CAD build for the part. Positions are in the model's coordinates, mm. A direction names the side the tool comes from. Give positions to 0.01 mm unless a question says otherwise; leave off trailing zeros. Loops run counter-clockwise (first coordinate to the right, second up) from the corner with the lowest first, then second, coordinate; pieces in that order, holes last.
Item 1: Which spindle directions (+Z, -Z, +X, -X, +Y, -Y) get a long thin tool onto all of the face, cutting with end or side? Do faces 4 (the flat face through (-24, 10.22, 1)), 5 (the flat face through (20, -9.12, 1)), 6 (the flat face through (0, 16.24, 14)). Say none if no direction does.
Item 2: Saw through at A-A on x = 25.05. Give the cut face in (y, z), plus the area to 3 significant figures.
Item 3: Saw through at C-C on y = 0. Give the cut face in (x, z).
Item 4: Saw through at B-B on z = 16.5. Give the cut face in (x, y), plus the area to 3 significant figures.
Item 5: Mould opens along Z. For faces 1 (the cylindrical face through (9.48, 17.38, 22.57)), 2 (the flat face through (-26, -12, 14)), 3 (the flat face through (0, 17, 25.4)) say: released by +Z, released by -Z, zero draft, split by the parting line, or undercut.
Item 6: Drop flat-ended pins along their axis: P1, Ø0.7, axis at x = -19.5, z = 1.5, coming from the -Y side; P2, Ø2.5, axis at x = -25.5, z = 11, coming from the +Y side; P3, Ø10, axis at x = 9, z = 17.5, coming from the -Y side. Give the stop position or say it passes through.
Item 7: Probe probe 1 along X at (y, z) = (17.6, 7.14); probe 2 along X at (y, z) = (-13.65, 19.14); probe 3 along Z at (x, y) = (8.5, 16.5). List the from-to ranges inside material, lowest first.
Item 8: Saw through at D-D on z = 10.25. Give the cut face in (x, y).
from build123d import *

# Parameters (mm, degrees)
BOSS_EXTRUDE1_DEPTH = 2.2
SKETCH1_3_W         = 42.3
SKETCH1_3_H         = 2.24
BOSS_EXTRUDE2_DEPTH = 25.4
SKETCH1_4_W         = 8.8
SKETCH1_4_H         = 2.28
BOSS_EXTRUDE3_DEPTH = 25.3
FILLET13_R          = 3
FILLET14_R          = 3
FILLET15_R          = 3
FILLET16_R          = 3
FILLET18_R          = 3
FILLET19_R          = 3
FILLET20_R          = 3
FILLET21_R          = 3
FILLET24_R          = 2.36
FILLET25_R          = 2.36
FILLET26_R          = 2.2
SKETCH2_R           = 2
CUT_EXTRUDE1_DEPTH  = 10
SKETCH3_R           = 1.5
CUT_EXTRUDE2_DEPTH  = 10
SKETCH4_R           = 1.5
CUT_EXTRUDE3_DEPTH  = 10


with BuildPart() as part:
    # Sketch1 → Boss-Extrude1 (new body)
    with BuildSketch(Plane.XY):
        Polygon((21.15, 16.24), (-21.15, 16.24), (-21.15, 10.22), (-21.15, -9.12), (-18.4, -9.12), (18.4, -9.12), (21.15, -9.12), (21.15, 10.22), align=None)
        with BuildLine():
            Line((-4.349812535, -18.48), (13.96, -18.48))
            ThreePointArc((13.96, -18.48), (17.099554108, -17.179554108), (18.4, -14.04))
            Line((18.4, -14.04), (18.4, -9.12))
            Line((18.4, -9.12), (-18.4, -9.12))
            Line((-18.4, -9.12), (-18.4, -14.04))
            ThreePointArc((-18.4, -14.04), (-17.099554108, -17.179554108), (-13.96, -18.48))
            Line((-13.96, -18.48), (-4.349812535, -18.48))
        make_face()
        Polygon((-21.15, -9.12), (-21.15, 10.22), (-29.95, 10.22), (-29.95, -12), (-21.15, -12), align=None)
        Polygon((29.95, 10.22), (21.15, 10.22), (21.15, -9.12), (21.15, -12), (29.95, -12), align=None)
    extrude(amount=BOSS_EXTRUDE1_DEPTH)

    # Sketch1<3> → Boss-Extrude2 (add)
    with BuildSketch(Plane.XY):
        with Locations((0, 17.36)):
            Rectangle(SKETCH1_3_W, SKETCH1_3_H)
    extrude(amount=BOSS_EXTRUDE2_DEPTH)

    # Sketch1<4> → Boss-Extrude3 (add)
    with BuildSketch(Plane.XY):
        with Locations((-25.55, -13.14)):
            Rectangle(SKETCH1_4_W, SKETCH1_4_H)
        with Locations((25.55, -13.14)):
            Rectangle(SKETCH1_4_W, SKETCH1_4_H)
    extrude(amount=BOSS_EXTRUDE3_DEPTH)

    # Fillet13
    fillet13_edges = [part.edges().sort_by_distance(p)[0] for p in [
        (-21.15, -13.14, 25.3),
    ]]
    fillet(fillet13_edges, radius=FILLET13_R)

    # Fillet14
    fillet14_edges = [part.edges().sort_by_distance(p)[0] for p in [
        (-29.95, -13.14, 25.3),
    ]]
    fillet(fillet14_edges, radius=FILLET14_R)

    # Fillet15
    fillet15_edges = [part.edges().sort_by_distance(p)[0] for p in [
        (29.95, -13.14, 25.3),
    ]]
    fillet(fillet15_edges, radius=FILLET15_R)

    # Fillet16
    fillet16_edges = [part.edges().sort_by_distance(p)[0] for p in [
        (21.15, -13.14, 25.3),
    ]]
    fillet(fillet16_edges, radius=FILLET16_R)

    # Fillet18
    fillet18_edges = [part.edges().sort_by_distance(p)[0] for p in [
        (21.15, 17.36, 25.4),
    ]]
    fillet(fillet18_edges, radius=FILLET18_R)

    # Fillet19
    fillet19_edges = [part.edges().sort_by_distance(p)[0] for p in [
        (-21.15, 17.36, 25.4),
    ]]
    fillet(fillet19_edges, radius=FILLET19_R)

    # Fillet20
    fillet20_edges = [part.edges().sort_by_distance(p)[0] for p in [
        (29.95, 10.22, 1.1),
    ]]
    fillet(fillet20_edges, radius=FILLET20_R)

    # Fillet21
    fillet21_edges = [part.edges().sort_by_distance(p)[0] for p in [
        (-29.95, 10.22, 1.1),
    ]]
    fillet(fillet21_edges, radius=FILLET21_R)

    # Fillet24
    fillet24_edges = [part.edges().sort_by_distance(p)[0] for p in [
        (-25.55, -14.28, 0),
    ]]
    fillet(fillet24_edges, radius=FILLET24_R)

    # Fillet25
    fillet25_edges = [part.edges().sort_by_distance(p)[0] for p in [
        (25.55, -14.28, 0),
    ]]
    fillet(fillet25_edges, radius=FILLET25_R)

    # Fillet26
    fillet26_edges = [part.edges().sort_by_distance(p)[0] for p in [
        (0, 18.48, 0),
    ]]
    fillet(fillet26_edges, radius=FILLET26_R)

    # Sketch2 → Cut-Extrude1 (cut)
    with BuildSketch(Plane.XZ.offset(14.28)):
        with Locations(Location((25.05, 19.14, 0), (0, 0, 270))):
            Circle(SKETCH2_R)
        with Locations(Location((25.05, 9.1, 0), (0, 0, 270))):
            Circle(SKETCH2_R)
        with Locations(Location((-25.15, 19.14, 0), (0, 0, 270))):
            Circle(SKETCH2_R)
        with Locations(Location((-25.15, 9.1, 0), (0, 0, 270))):
            Circle(SKETCH2_R)
    extrude(amount=-CUT_EXTRUDE1_DEPTH, mode=Mode.SUBTRACT)

    # Sketch3 → Cut-Extrude2 (cut)
    with BuildSketch(Plane(origin=(0, 18.48, 0), x_dir=(1, 0, 0), z_dir=(0, 1, 0))):
        with Locations(Location((9.03, -14.14, 0), (0, 0, 270))):
            Circle(SKETCH3_R)
        with Locations(Location((9.03, -7.14, 0), (0, 0, 270))):
            Circle(SKETCH3_R)
        with Locations(Location((16.03, -14.14, 0), (0, 0, 270))):
            Circle(SKETCH3_R)
        with Locations(Location((9.03, -21.14, 0), (0, 0, 270))):
            Circle(SKETCH3_R)
        with Locations(Location((2.03, -14.14, 0), (0, 0, 270))):
            Circle(SKETCH3_R)
        with Locations(Location((-9.605424329, -14.14, 0), (0, 0, 270))):
            Circle(SKETCH3_R)
        with Locations(Location((-9.605424329, -7.14, 0), (0, 0, 270))):
            Circle(SKETCH3_R)
        with Locations(Location((-2.605424329, -14.14, 0), (0, 0, 270))):
            Circle(SKETCH3_R)
        with Locations(Location((-9.605424329, -21.14, 0), (0, 0, 270))):
            Circle(SKETCH3_R)
        with Locations(Location((-16.605424329, -14.14, 0), (0, 0, 270))):
            Circle(SKETCH3_R)
    extrude(amount=-CUT_EXTRUDE2_DEPTH, mode=Mode.SUBTRACT)

    # Sketch4 → Cut-Extrude3 (cut)
    with BuildSketch(Plane(origin=(0, 0, 0), x_dir=(-1, 0, 0), z_dir=(0, 0, -1))):
        with Locations((-7, 0)):
            Circle(SKETCH4_R)
        with Locations((0, 7)):
            Circle(SKETCH4_R)
        with Locations((7, 0)):
            Circle(SKETCH4_R)
        with Locations((0, -7)):
            Circle(SKETCH4_R)
        Circle(SKETCH4_R)
    extrude(amount=-CUT_EXTRUDE3_DEPTH, mode=Mode.SUBTRACT)


solid = part.part
Results below:
1. face 4: +Z, -Z, -X, +Y
1. face 5: +Z, -Z, -Y
1. face 6: +Z, +X, -X, -Y
2. outline: (-14.28, 2.36) arc R2.36 ccw to (-11.92, 0) - (10.22, 0) - (10.22, 2.2) - (-12, 2.2) - (-12, 7.1) - (-14.28, 7.1) - close; (-14.28, 11.1) - (-12, 11.1) - (-12, 17.14) - (-14.28, 17.14) - close; (-14.28, 21.14) - (-12, 21.14) - (-12, 25.3) - (-14.28, 25.3) - close
2. area: 87.1 mm2
3. outline: (-29.95, 0) - (-8.5, 0) - (-8.5, 2.2) - (-29.95, 2.2) - close; (-5.5, 0) - (-1.5, 0) - (-1.5, 2.2) - (-5.5, 2.2) - close; (1.5, 0) - (5.5, 0) - (5.5, 2.2) - (1.5, 2.2) - close; (8.5, 0) - (29.95, 0) - (29.95, 2.2) - (8.5, 2.2) - close
4. outline: (-29.95, -14.28) - (-21.15, -14.28) - (-21.15, -12) - (-29.95, -12) - close; (-21.15, 16.24) - (21.15, 16.24) - (21.15, 18.48) - (-21.15, 18.48) - close; (21.15, -14.28) - (29.95, -14.28) - (29.95, -12) - (21.15, -12) - close
4. area: 135 mm2
5. face 1: undercut
5. face 2: zero draft
5. face 3: released by +Z
6. P1: stops at y = -9.12
6. P2: stops at y = -12
6. P3: stops at y = 16.24
7. probe 1: x = -21.15 to -11.11, -8.11 to 7.53, 10.53 to 21.15
7. probe 2: x = -29.95 to -27.15, -23.15 to -21.15, 21.15 to 23.05, 27.05 to 29.95
7. probe 3: z = 0.01 to 5.74, 8.54 to 12.74, 15.54 to 19.74, 22.54 to 25.4
8. outline: (-29.95, -14.28) - (-26.79, -14.28) - (-26.79, -12) - (-29.95, -12) - close; (-23.51, -14.28) - (-21.15, -14.28) - (-21.15, -12) - (-23.51, -12) - close; (-21.15, 16.24) - (21.15, 16.24) - (21.15, 18.48) - (-21.15, 18.48) - close; (21.15, -14.28) - (23.41, -14.28) - (23.41, -12) - (21.15, -12) - close; (26.69, -14.28) - (29.95, -14.28) - (29.95, -12) - (26.69, -12) - close
